CAD build for the part. Positions are in the model's coordinates, mm. Face numbers are marked on the shaded views. A direction names the side the tool comes from. Coordinates: 2 decimals unless noted, no trailing zeros. Write each loop counter-clockwise with the first axis right and the second up, starting at its lowest first coordinate (ties: lowest second). Pieces come first, ordered by that corner, then holes. Notation, with made-up numbers: (55, -34) -> (70, -34) arc R28 ccw to (70, -12) -> close; hole circle Ø4 at (-10.5, 85.5). An arc over 180 degrees is marked (long way). Answer as CSV lines item,"result".
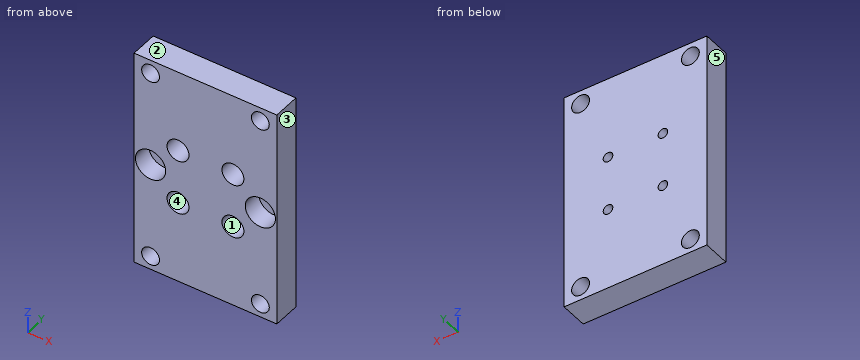
```python
from build123d import *

# Parameters (mm, degrees)
F0_W     = 52
F0_H     = 80
F0_R     = 3.25
F0_R_2   = 1.75
F1_DEPTH = 10
F2_R     = 5.5
F3_DEPTH = 7
F4_R     = 4
F5_DEPTH = 7


with BuildPart() as f1:
    # F0 (on Front) → F1 (new body)
    with BuildSketch(Plane.XZ):
        Rectangle(F0_W, F0_H)
        with Locations((-20, -35)):
            Circle(F0_R, mode=Mode.SUBTRACT)
        with Locations((-10, -10)):
            Circle(F0_R_2, mode=Mode.SUBTRACT)
        with Locations((20, -35)):
            Circle(F0_R, mode=Mode.SUBTRACT)
        with Locations((10, -10)):
            Circle(F0_R_2, mode=Mode.SUBTRACT)
        with Locations((-10, 10)):
            Circle(F0_R_2, mode=Mode.SUBTRACT)
        with Locations((-20, 35)):
            Circle(F0_R, mode=Mode.SUBTRACT)
        with Locations((10, 10)):
            Circle(F0_R_2, mode=Mode.SUBTRACT)
        with Locations((20, 35)):
            Circle(F0_R, mode=Mode.SUBTRACT)
    extrude(amount=F1_DEPTH)

    # F2 (on face) → F3 (cut)
    with BuildSketch(Plane.XZ.offset(10)):
        with Locations((-20, 0)):
            Circle(F2_R)
        with Locations((20, 0)):
            Circle(F2_R)
    extrude(amount=-F3_DEPTH, mode=Mode.SUBTRACT)

    # F4 (on face) → F5 (cut)
    with BuildSketch(Plane.XZ.offset(10)):
        with Locations((-10, 10)):
            Circle(F4_R)
        with Locations((10, 10)):
            Circle(F4_R)
        with Locations((-10, -10)):
            Circle(F4_R)
        with Locations((10, -10)):
            Circle(F4_R)
    extrude(amount=-F5_DEPTH, mode=Mode.SUBTRACT)


solid = f1.part
```
Item 1: Saw through at D-D on z = -10. Give the cut face in (x, y).
Answer below:
outline,"(-26, -10) -> (-14, -10) -> (-14, -3) -> (-11.75, -3) -> (-11.75, 0) -> (-26, 0) -> close; (-8.25, -3) -> (-6, -3) -> (-6, -10) -> (6, -10) -> (6, -3) -> (8.25, -3) -> (8.25, 0) -> (-8.25, 0) -> close; (11.75, -3) -> (14, -3) -> (14, -10) -> (26, -10) -> (26, 0) -> (11.75, 0) -> close"
Item 2: Two-plate mould, pull along Z, no slides. Class the marked faces 1, 2 and 3: pulls with the +Z half, pulls with the -Z half, needs draft (parallel to the pull), parting line crosses it, or undercut.
Answer below:
face 1,"undercut"
face 2,"pulls with the +Z half"
face 3,"needs draft"
Item 3: 3-axis set-ups, long thin cutter, end or side, ignore diameter. For the marked faces 4 and 5: which of +Z, -Z, +X, -X, +Y, -Y reach the whole face in a straight line?
Answer below:
face 4,"-Y"
face 5,"+Z, -Z, -X, +Y, -Y"
Item 4: Saw through at B-B on z = 35. Give the cut face in (x, y), and give its area (3 significant figures).
Answer below:
outline,"(-26, -10) -> (-23.25, -10) -> (-23.25, 0) -> (-26, 0) -> close; (-16.75, -10) -> (16.75, -10) -> (16.75, 0) -> (-16.75, 0) -> close; (23.25, -10) -> (26, -10) -> (26, 0) -> (23.25, 0) -> close"
area,"390 mm2"
Item 5: Saw through at A-A on x = 20. Give the cut face in (y, z), and give its area (3 significant figures).
Answer below:
outline,"(-10, -40) -> (0, -40) -> (0, -38.25) -> (-10, -38.25) -> close; (-10, -31.75) -> (0, -31.75) -> (0, 31.75) -> (-10, 31.75) -> (-10, 5.5) -> (-3, 5.5) -> (-3, -5.5) -> (-10, -5.5) -> close; (-10, 38.25) -> (0, 38.25) -> (0, 40) -> (-10, 40) -> close"
area,"593 mm2"
Item 6: Flat gauge pins, fed straight in: pin 1 (2.5 mm diameter, centred on x = -9.5, z = 8.5, fed in from -Y); pin 2 (10 mm diameter, centred on x = -2, z = 9, fed in from +Y). Where does each tip first touch, or does it go through?
Answer below:
pin 1,"stops at y = -3"
pin 2,"stops at y = 0"
Item 7: Wall check: line 1 (Z direction, x = 10, y = -1); line 2 (X direction, y = -1, z = -10); line 3 (Z direction, x = -20, y = -1.75). Give the ranges that are in metal, low to high. Write a range as from..to.
Answer below:
line 1,"z = -40..-11.75, -8.25..8.25, 11.75..40"
line 2,"x = -26..-11.75, -8.25..8.25, 11.75..26"
line 3,"z = -40..-38.25, -31.75..31.75, 38.25..40"
Item 8: Saw through at C-C on y = -4.25. State how many separate pieces and enclosed holes the cut face has, and give its area (3 significant figures).
Answer below:
separate pieces,"1"
enclosed holes,"10"
area,"3,640 mm2"
